Work out the finished part from the listing and answer in its coordinate system (mm). Give positions to 0.01 mm unless a question says otherwise; leave off trailing zeros. Order: outer loops, then holes, each group sorted by start corner. A loop starts at its lowest first (then second) coordinate and runs counter-clockwise, first axis right, second up. Notation, with made-up numbers: M 72.25,10.25 L 83.25,10.25 A29 cw 83.25,48.25 Z; hole C 34,16 d3. An arc over 180 degrees is marked long. One line per item, written item: value.
from build123d import *

# Parameters (mm, degrees)
CROQUIS1_R              = 3
SALIENTE_EXTRUIR1_DEPTH = 3


with BuildPart() as part:
    # Croquis1 → Saliente-Extruir1 (new body)
    with BuildSketch(Plane.XY):
        with BuildLine():
            Line((0, -60), (0, 0))
            ThreePointArc((0, 0), (17.5, 17.5), (35, 0))
            Line((35, 0), (35, -60))
            Line((35, -60), (30, -60))
            Line((30, -60), (30, -57))
            Line((30, -57), (25, -57))
            Line((25, -57), (25, -60))
            Line((25, -60), (20, -60))
            Line((20, -60), (20, -57))
            Line((20, -57), (15, -57))
            Line((15, -57), (15, -60))
            Line((15, -60), (10, -60))
            Line((10, -60), (10, -57))
            Line((10, -57), (5, -57))
            Line((5, -57), (5, -60))
            Line((5, -60), (0, -60))
        make_face()
        with Locations((17.5, 0)):
            Circle(CROQUIS1_R, mode=Mode.SUBTRACT)
    extrude(amount=SALIENTE_EXTRUIR1_DEPTH)


solid = part.part
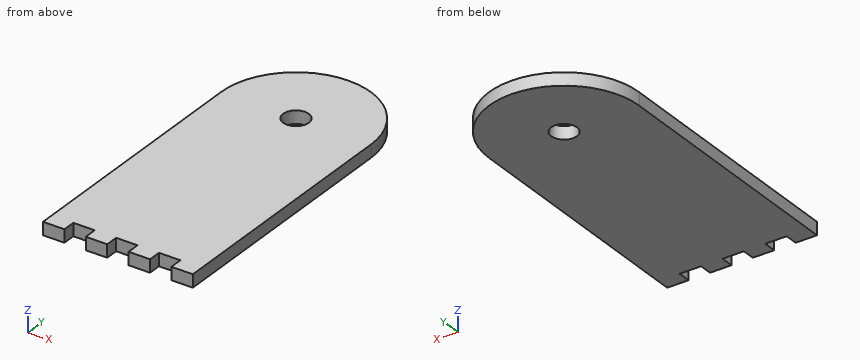
(1) Section B-B, the plane z = 1.95 is taken. Give the vertices of the cut face in (x, y).
Findings:
outline: M 0,-60 L 5,-60 L 5,-57 L 10,-57 L 10,-60 L 15,-60 L 15,-57 L 20,-57 L 20,-60 L 25,-60 L 25,-57 L 30,-57 L 30,-60 L 35,-60 L 35,0 A17.5 ccw 0,0 Z; hole C 17.5,0 d6
(2) Section A-A, the plane x = 17.5 is taken. Give the vertices of the cut face in (y, z), then the cut area to 4 significant figures.
Findings:
outline: M -57,0 L -3,0 L -3,3 L -57,3 Z; M 3,0 L 17.5,0 L 17.5,3 L 3,3 Z
area: 205.5 mm^2
(3) Given P1, Ø1.5, axis at x = 18.5, z = 1.5, coming from the -Y side; P2, Ø5, axis at x = 17.5, y = 0, coming from the -Z side, each flat-ended and moving along its own axis, determine where each tip first touches the part or whether it passes through.
Findings:
P1: stops at y = -57
P2: passes through
(4) Find the intervals of material crossed by probe 1 along Y at (x, z) = (17.5, 1.3); probe 2 along X at (y, z) = (1, 0.95); probe 3 along Y at (x, z) = (28.5, 0.7), in increasing order. Write a range as from..to.
Findings:
probe 1: y = -57..-3, 3..17.5
probe 2: x = 0.03..14.67, 20.33..34.97
probe 3: y = -57..13.61
(5) Section C-C, the plane x = 24 is taken. Give the vertices of the cut face in (y, z), then the cut area to 3 significant figures.
Findings:
outline: M -60,0 L 16.25,0 L 16.25,3 L -60,3 Z
area: 229 mm^2
